```python
from build123d import *

# Parameters (mm, degrees)
F_1_FR_W        = 43.350723316
F_1_FR_H        = 38.259713105
EXTRUDE_1_DEPTH = 20
EXTRUDE_1_TAPER = 20
OTHER_START     = -1
OTHER_1_DEPTH   = 45
OTHER_START_2   = 7.279404685
OTHER_1_2_DEPTH = 28.791913946
OTHER_START_3   = -35.822740595
OTHER_1_3_DEPTH = 32.835074171


with BuildPart() as part:
    # Эскиз1_fr → Бобышка-Вытянуть1 (new body)
    with BuildSketch(Plane.XY):
        with Locations((21.675361658, -19.129856553)):
            Rectangle(F_1_FR_W, F_1_FR_H)
    extrude(amount=EXTRUDE_1_DEPTH, taper=EXTRUDE_1_TAPER)

    # Заменить грань1: read off the stored shape, not the designer's step
    # Заменить грань1 outline → Заменить грань1 (cut)
    with BuildSketch(Plane.YZ.offset(OTHER_START)):
        with BuildLine():
            Line((0, 0), (-2.987666524, 8.208546313))
            add(Edge.make_bspline(
                [(-2.987666524, 8.208546313), (-8.870550538, 9.578826995), (-19.207758762, -1.740918138), (-30.435430933, 4.410138177), (-35.822740495, 6.695527216)],
                knots=[0.134570032, 0.134570032, 0.134570032, 0.134570032, 0.484609084, 0.79490495, 0.79490495, 0.79490495, 0.79490495], degree=3))
            Line((-35.822740495, 6.695527216), (-38.259713105, 0))
            Line((-38.259713105, 0), (0, 0))
        make_face()
    extrude(amount=OTHER_1_DEPTH, mode=Mode.SUBTRACT)

    # Other 1 2 outline → Other 1 2 (add)
    with BuildSketch(Plane.YZ.offset(OTHER_START_2)):
        with BuildLine():
            Line((-7.279404685, 20), (-9.965660529, 27.380427273))
            add(Edge.make_bspline(
                [(-9.965660529, 27.380427273), (-12.601354954, 25.979247634), (-18.69943354, 22.300628932), (-25.092854244, 24.416589038), (-28.802415021, 25.983712933)],
                knots=[0.320991938, 0.320991938, 0.320991938, 0.320991938, 0.484609084, 0.701285336, 0.701285336, 0.701285336, 0.701285336], degree=3))
            Line((-28.802415021, 25.983712933), (-30.980308419, 20))
            Line((-30.980308419, 20), (-7.279404685, 20))
        make_face()
    extrude(amount=OTHER_1_2_DEPTH)

    # Other 1 3 outline → Other 1 3 (cut)
    with BuildSketch(Plane(origin=(0, 0, 0), x_dir=(1, 0, 0), z_dir=(0, 1, 0)).offset(OTHER_START_3)):
        Polygon((9.965660529, -27.380427273), (7.279404685, -20), (7.279404685, -29), (10.555136794, -29), align=None)
        Polygon((33.385062787, -27.380427273), (32.795586522, -29), (36.071318631, -29), (36.071318631, -20), align=None)
    extrude(amount=OTHER_1_3_DEPTH, mode=Mode.SUBTRACT)


solid = part.part
```
The model under review builds one solid part; all positions refer to its coordinate system, in mm. Give positions to 0.01 mm unless a question says otherwise; leave off trailing zeros. Write each loop counter-clockwise with the first axis right and the second up, starting at its lowest first coordinate (ties: lowest second). Pieces come first, ordered by that corner, then holes. Notation, with made-up numbers: (73.25, 58) - (121.25, 58) arc R12 ccw to (121.25, 78) - close; hole circle Ø9 at (3, 51). An arc over 180 degrees is marked (long way). Answer in a Markdown table with one row per item. Add a question column.
1. We need section B-B on z = 15.25. Write out the cut boundary in (x, y).
2. Wall thickness on line 1 along Z through (x, y) = (16.5, -12); line 2 along Y through (x, z) = (14.5, 11.75); line 3 along X through (y, z) = (-25, 13): over which ranges is each line inside the solid? List them lowest first. Write a range as [from, to].
3. Insertion check: P1, Ø12, axis at x = 31.5, y = -11, coming from the -Z side; P2, Ø4, axis at y = -27.5, z = 13.5, coming from the -X side; P3, Ø10, axis at x = 34, z = 10, coming from the -Y side; P4, Ø3, axis at y = -27.5, z = 9.5, coming from the -X side. Each pin has a flat end and moves straight along its axis. Give the tip position at first contact, or say it passes through.
4. We need section A-A on z = 11.5. Write out the cut boundary in (x, y), then the cut area to 3 significant figures.
Ans:
| question | item | result |
|---|---|---|
| 1 | outline | (5.55, -32.71) - (37.8, -32.71) - (37.8, -5.55) - (5.55, -5.55) - close |
| 2 | line 1 | z = [6.06, 26.28] |
| 2 | line 2 | y = [-33.98, -4.28] |
| 2 | line 3 | x = [4.73, 38.62] |
| 3 | P1 | stops at z = 3.48 |
| 3 | P2 | stops at x = 4.19 |
| 3 | P3 | stops at y = -35.82 |
| 3 | P4 | stops at x = 2.91 |
| 4 | outline | (4.19, -34.07) - (39.17, -34.07) - (39.17, -4.19) - (4.19, -4.19) - close |
| 4 | area | 1,050 mm^2 |
